Geometry: final body of the model. Coordinates: model frame, mm. Face numbers are marked on the shaded views. Round coordinates to 2 decimals unless told otherwise and drop trailing zeros. Loops run counter-clockwise (first coordinate to the right, second up) from the corner with the lowest first, then second, coordinate; pieces in that order, holes last. Notation, with made-up numbers: (-9.5, -19.5) - (38.5, -19.5) arc R21 cw to (38.5, 16.5) - close; hole circle Ø5 at (88.25, 55). An arc over 180 degrees is marked (long way). Return JSON: item names as keys, results as strings. Group by question number.
1. Section B-B on x = 302. Return loops of the section in (y, z).
2. Section A-A on y = -20.5. Return loops of the section in (x, z).
3. Material intervals for probe 1 along Y at (x, z) = (348, -34.5); probe 2 along Z at (x, y) = (14, -33); probe 3 along Z at (x, y) = (-75, 11), sorted ascending.
4. First-contact query: pin 1 Ø6 at (y, z) = (-40, -31) entering from +X; pin 2 Ø16 at (x, z) = (354.82, -26.79) entering from +Y; pin 3 Ø5 at (x, y) = (206, -29) entering from -Z; pin 4 Ø3 at (x, y) = (220.5, -4) entering from -Z. Flat tips, straight axial feed; report the tip coordinate or a pass-through.
5. Section C-C on y = -73. Return loops of the section in (x, z).
6. Draft query along Z for the marked faces 1 and 2. Return one class per face: +Z half, -Z half, draft (parallel to the pull), parting line (faces both ways), or undercut.
7. Section D-D on y = -45. Return loops of the section in (x, z), and give its area (3 significant figures).
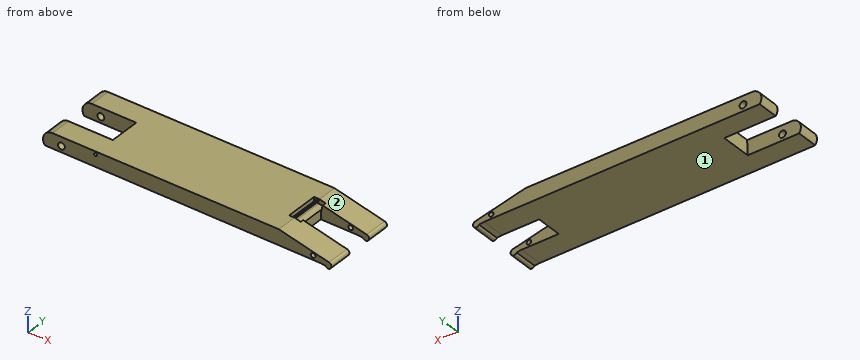
from build123d import *

# Parameters (mm, degrees)
F1_DEPTH      = 85
F2_W          = 140.1526774555
F2_H          = 71.5
F2_W_2        = 166.0307588987
F2_H_2        = 60
F3_DEPTH      = 60
F4_R          = 5
F5_DEPTH      = 115.001
F5_DEPTH_BACK = 55.001
F6_R          = 7.5
F7_DEPTH      = 120.751
F7_DEPTH_BACK = 49.251
F8_W          = 2.8015428152
F8_H          = 60
F9_DEPTH      = 10
F11_W         = 11.8633863517
F11_H         = 76.3498097658
F12_DEPTH     = 10
F13_R         = 2.5
F14_DEPTH     = 76.3498097658
F15_R         = 3.25
F16_DEPTH     = 20


# Not quite as in the source:
# - a feature of the source that left no trace in its solid (it failed there, or was rolled back) is left out
# - a feature names something its author has since deleted; it is built from what else it names


with BuildPart() as f1:
    # F0 (on Front) → F1 (new body, symmetric)
    with BuildSketch(Plane.XZ):
        with BuildLine():
            Line((279.3908679786, 0.7735525745), (-219.4691173488, 19.9851854498))
            ThreePointArc((-219.4691173488, 19.9851854498), (-237.9331597041, 9.3224734741), (-236.2868942017, -11.9355625752))
            Line((-236.2868942017, -11.9355625752), (370.8640205953, -36.8868572182))
            Line((370.8640205953, -36.8868572182), (382.0565363882, -38.6184028055))
            ThreePointArc((382.0565363882, -38.6184028055), (393.7122397041, -39.6064498563), (390.0009393692, -28.5133030266))
            Line((390.0009393692, -28.5133030266), (279.3908679786, 0.7735525745))
        make_face()
    extrude(amount=F1_DEPTH, both=True)

    # F2 (on face) → F3 (cut)
    with BuildSketch(Plane(origin=(0.44349793, 0, 11.5161148616), x_dir=(0.9992592725, 0, -0.0384825459), z_dir=(0.0384825459, 0, 0.9992592725))):
        with Locations((-192.4187466502, 0)):
            Rectangle(F2_W, F2_H)
        with Locations((373.3601896558, 0)):
            Rectangle(F2_W_2, F2_H_2)
    extrude(amount=-F3_DEPTH, mode=Mode.SUBTRACT)

    # F4 (on face) → F5 (cut, two sides)
    with BuildSketch(Plane(origin=(0, -30, 0), x_dir=(-1, 0, 0), z_dir=(0, 1, 0))) as f5_sk:
        with Locations((-354.8175990582, -26.7948582768)):
            Circle(F4_R)
    extrude(amount=F5_DEPTH, mode=Mode.SUBTRACT)
    extrude(f5_sk.sketch, amount=-F5_DEPTH_BACK, mode=Mode.SUBTRACT)

    # F6 (on face) → F7 (cut, two sides)
    with BuildSketch(Plane.XZ.offset(-35.75)) as f7_sk:
        with Locations((-199.6834129095, 0)):
            Circle(F6_R)
    extrude(amount=F7_DEPTH, mode=Mode.SUBTRACT)
    extrude(f7_sk.sketch, amount=-F7_DEPTH_BACK, mode=Mode.SUBTRACT)

    # F8 (on face) → F9 (cut)
    with BuildSketch(Plane(origin=(18.495209297, 0, 69.8523750243), x_dir=(0.9666885377, 0, -0.2559556038), z_dir=(0.2559556038, 0, 0.9666885377))):
        Polygon((270.5007791519, -37.1644198895), (284.1554284096, -37.1644198895), (284.1554284096, -30), (281.3538855944, -30), (281.3538855944, 30), (284.1554284096, 30), (284.1554284096, 39.305575192), (270.5007791519, 39.305575192), align=None)
        with Locations((282.754657002, 0)):
            Rectangle(F8_W, F8_H)
    extrude(amount=-F9_DEPTH, mode=Mode.SUBTRACT)

    # F11 (on face) → F12 (cut)
    with BuildSketch(Plane(origin=(0.44349793, 0, 11.5161148616), x_dir=(0.9992592725, 0, -0.0384825459), z_dir=(0.0384825459, 0, 0.9992592725))):
        with Locations((273.2224540287, 1.0649263859)):
            Rectangle(F11_W, F11_H)
    extrude(amount=-F12_DEPTH, mode=Mode.SUBTRACT)

    # F13 (on face) → F14 (join, through all)
    with BuildSketch(Plane.XZ.offset(-39.2398312688)):
        with Locations((274.223446846, -4.3092062697)):
            Circle(F13_R)
    extrude(amount=F14_DEPTH)

    # F15 (on face) → F16 (cut)
    with BuildSketch(Plane.XZ.offset(85)):
        with Locations((-124.1565719247, 9.9523849785)):
            Circle(F15_R)
    extrude(amount=-F16_DEPTH, mode=Mode.SUBTRACT)


solid = f1.part
Taken from the geometry:
{
 "1": {"outline": "(-85, -34.06) - (-30, -34.06) - (-30, -5.21) - (-85, -5.21) - close; (30, -34.06) - (85, -34.06) - (85, -5.21) - (30, -5.21) - close"},
 "2": {"outline": "(-123.07, -16.59) - (289.27, -33.53) - (290.08, -12.4) - (277.9, -9.18) - (267.15, -8.76) - (267.54, 1.23) - (-121.81, 16.22) - close; circle Ø5 at (274.22, -4.31); (279.28, -2.04) - (279.99, 0.62) - (279.39, 0.77) - close"},
 "3": {"probe 1": "-85 to -30, 30 to 85", "probe 2": "-22.22 to 10.99", "probe 3": "-18.56 to 14.42"},
 "4": {"pin 1": "x = 395.09", "pin 2": "y = 85", "pin 3": "z = -30.21", "pin 4": "z = -30.77"},
 "5": {"outline": "(-236.29, -11.94) - (370.86, -36.89) - (382.06, -38.62) arc R7 ccw (long way) to (390, -28.51) - (279.39, 0.77) - (-219.47, 19.99) arc R20 ccw to start; hole circle Ø15 at (-199.68, 0); hole circle Ø6.5 at (-124.16, 9.95); hole circle Ø10 at (354.82, -26.79)"},
 "6": {"face 1": "-Z half", "face 2": "+Z half"},
 "7": {"outline": "(-236.29, -11.94) - (370.86, -36.89) - (382.06, -38.62) arc R7 ccw (long way) to (390, -28.51) - (279.39, 0.77) - (-219.47, 19.99) arc R20 ccw to start; hole circle Ø15 at (-199.68, 0); hole circle Ø10 at (354.82, -26.79)", "area": "19,400 mm2"}
}
